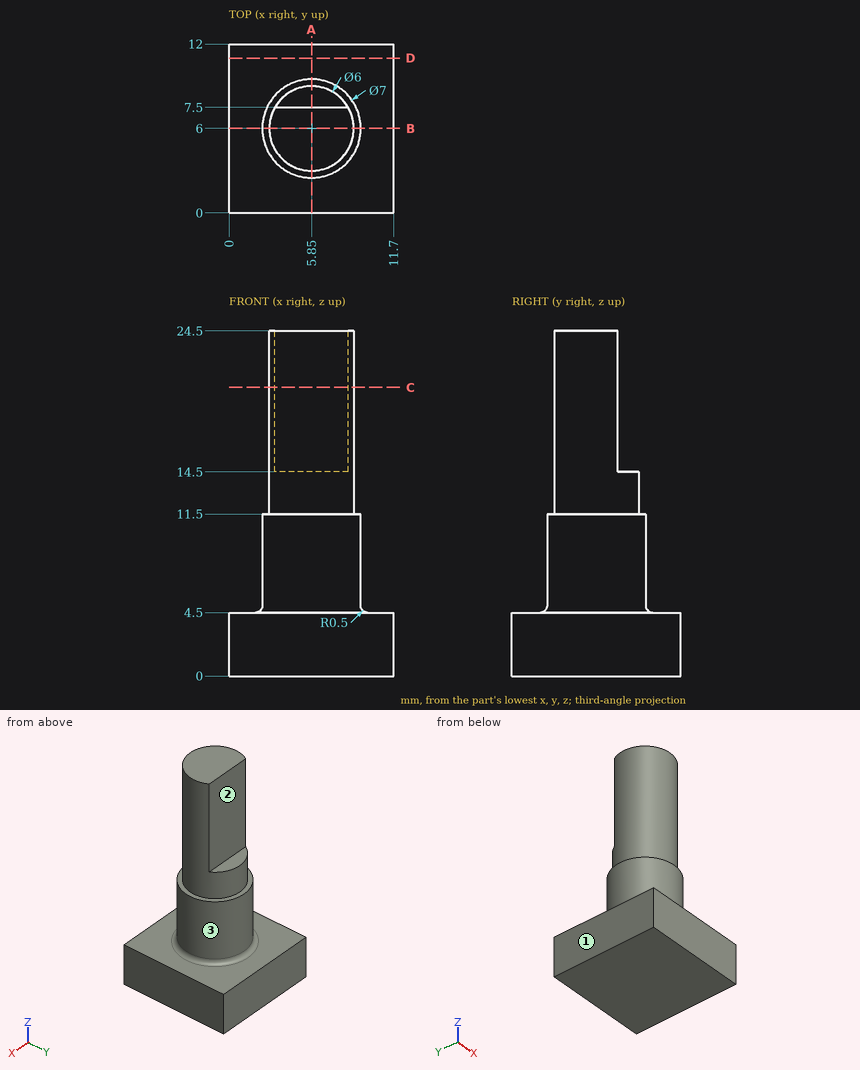
Drawing for the job (mm, zero at the part's lowest x, y, z). A direction names the side the tool comes from. Give positions to 0.01 mm unless a question says otherwise; leave off trailing zeros. Order: outer loops, then holes, each group sorted by start corner. A loop starts at its lowest first (then second) coordinate and runs counter-clockwise, first axis right, second up. Notation, with made-up numbers: M -33.5,82.5 L -1.5,82.5 A17 cw -1.5,86.5 Z; hole C 44,-5.5 d6. An arc over 180 degrees is marked long. Put each result on its own line as item: value. Start each with the question number.
(1) Saw through at A-A, the plane x = 5.85. Write the cut outline in (y, z).
(2) Saw through at B-B, the plane y = 6. Write the cut outline in (x, z).
(3) Saw through at C-C, the plane z = 20.5. Write the cut outline in (x, y).
(4) Saw through at D-D, the plane y = 11. Write the cut outline in (x, z).
(5) Which spindle directions (+Z, -Z, +X, -X, +Y, -Y) get a long thin tool onto all of the face, cutting with end or side? Do the marked faces 1, 2 and 3. Say none if no direction does.
(6) Flat gauge pins, fed straight in: pin 1 Ø4 at (x, z) = (6, 19) entering from +Y; pin 2 Ø4 at (x, z) = (7.5, 8.5) entering from +Y; pin 3 Ø1.6 at (x, y) = (5.5, 8.5) entering from +Z. Where does each tip first touch, or does it go through?
(7) Drill centre lines: line 1 along Z through (x, y) = (8, 8.25); line 2 along Z through (x, y) = (11, 1.25); line 3 along Y through (x, z) = (5.75, 20). Where is each one in solid material? Low to high.
Check result:
1. outline: M 0,0 L 12,0 L 12,4.5 L 10,4.5 A0.5 cw 9.5,5 L 9.5,11.5 L 9,11.5 L 9,14.5 L 7.5,14.5 L 7.5,24.5 L 3,24.5 L 3,11.5 L 2.5,11.5 L 2.5,5 A0.5 cw 2,4.5 L 0,4.5 Z
2. outline: M 0,0 L 11.7,0 L 11.7,4.5 L 9.85,4.5 A0.5 cw 9.35,5 L 9.35,11.5 L 8.85,11.5 L 8.85,24.5 L 2.85,24.5 L 2.85,11.5 L 2.35,11.5 L 2.35,5 A0.5 cw 1.85,4.5 L 0,4.5 Z
3. outline: M 3.25,7.5 A3 ccw long 8.45,7.5 Z
4. outline: M 0,0 L 11.7,0 L 11.7,4.5 L 0,4.5 Z
5. face 1: +Z, -Z, -X, +Y, -Y
5. face 2: +Z, +X, -X, +Y
5. face 3: +Z
6. pin 1: stops at y = 7.5
6. pin 2: stops at y = 9.5
6. pin 3: stops at z = 14.5
7. line 1: z = 0 to 11.5
7. line 2: z = 0 to 4.5
7. line 3: y = 3 to 7.5
